Build history of the part. All positions in model axes, mm. A direction names the side the tool comes from. Coordinates: 2 decimals unless noted, no trailing zeros. Loops run counter-clockwise (first coordinate to the right, second up) from the corner with the lowest first, then second, coordinate; pieces in that order, holes last.
Item 1: Flat gauge pins, fed straight in: pin 1 (3 mm diameter, centred on y = 12.5, z = 1, fed in from +X); pin 2 (11.5 mm diameter, centred on x = 0, y = 15, fed in from +Z); pin 3 (1.5 mm diameter, centred on x = 18.5, z = 4.5, fed in from -Y); pin 4 (3 mm diameter, centred on x = -9.5, z = 2.5, fed in from +Y). Where does each tip first touch, or does it go through?
Item 2: Cut at D-D (x = -23.5). List the corners of the cut face in (y, z).
Item 3: 3-axis set-ups, long thin cutter, end or side, ignore diameter. For faces 1 (the face through (0, 0, 0)), 2 (the face through (26, 0, 2)): which of +Z, -Z, +X, -X, +Y, -Y reach the whole face in a straight line?
Item 4: Drill centre lines: line 1 along Y through (x, z) = (0, 2); line 2 along X through (y, z) = (-17, 3.45); line 3 along Y through (x, z) = (-3.5, 0.35). Where is each one in solid material? Low to high.
Item 5: Cut at A-A (z = 2.15). List the corners of the cut face in (x, y), and give its area (3 significant figures).
Item 6: Cut at B-B (x = 0). List the corners of the cut face in (y, z), and give its area (3 significant figures).
Item 7: Cut at C-C (y = 0). List the corners of the cut face in (x, z), and give its area (4 significant figures).
Item 8: Mould opens along Y. For faces 3 (the face through (0, 0, 5)), 4 (the face through (-29.97, -1.32, 2.46)), 5 (the face through (15.76, -18.41, 2.46)) say: released by +Y, released by -Y, zero draft, split by the parting line, or undercut.
Autodesk Fusion 360 part; units mm, degrees
sketch "Sketch1" plane through (0, 0, 0) normal (0, 0, 1) x (1, 0, 0)
  circle A0 centre (0, -15) radius 5
  circle A1 centre (0, 15) radius 5
  line L0 (26.5, 0) -> (27.807, 0) construction
  circle A2 centre (0, 0) radius 30
  line L1 (22.25, 0) -> (27.7377, 0) construction
  arc A3 (18.3848, 18.3848) -> (15.7331, 15.7331) centre (17.059, 17.059) ccw
  arc A4 (-15.7331, 15.7331) -> (-18.3848, 18.3848) centre (-17.059, 17.059) ccw
  arc A5 (15.7331, -15.7331) -> (18.3848, -18.3848) centre (17.059, -17.059) ccw
  arc A6 (-18.3848, -18.3848) -> (-15.7331, -15.7331) centre (-17.059, -17.059) ccw
  arc A7 (-15.7331, 15.7331) -> (-15.7331, -15.7331) centre (0, 0) ccw
  arc A8 (15.7331, -15.7331) -> (15.7331, 15.7331) centre (0, 0) ccw
  arc A9 (-18.3848, 18.3848) -> (-18.3848, -18.3848) centre (0, 0) ccw
  arc A10 (18.3848, -18.3848) -> (18.3848, 18.3848) centre (0, 0) ccw
  dimension "d4" = 15
  dimension "d5" = 10
  dimension "d11" = 60
  dimension "d12" = 52
  dimension "d16" = 44.5
  dimension "d17" = 3.75
extrude "Extrude1" add sketch "Sketch1" along normal blind 5
Filled sheet:
1. pin 1: stops at x = 27.91
1. pin 2: stops at z = 5
1. pin 3: stops at y = -24.19
1. pin 4: stops at y = 28.91
2. outline: (-18.65, 0) - (-11.12, 0) - (-11.12, 5) - (-18.65, 5) - close; (11.12, 0) - (18.65, 0) - (18.65, 5) - (11.12, 5) - close
3. face 1: -Z, +X, -X, +Y, -Y
3. face 2: +Z, -Z
4. line 1: y = -30 to -20, -10 to 10, 20 to 30
4. line 2: x = -24.72 to -19.67, -15.18 to -4.58, 4.58 to 15.18, 19.67 to 24.72
4. line 3: y = -29.8 to -18.57, -11.43 to 11.43, 18.57 to 29.8
5. outline: circle Ø60 at (0, 0); hole (-18.38, -18.38) arc R1.88 ccw to (-15.73, -15.73) arc R22.25 cw to (-15.73, 15.73) arc R1.88 ccw to (-18.38, 18.38) arc R26 ccw to start; hole circle Ø10 at (0, -15); hole circle Ø10 at (0, 15); hole (15.73, -15.73) arc R1.88 ccw to (18.38, -18.38) arc R26 ccw to (18.38, 18.38) arc R1.88 ccw to (15.73, 15.73) arc R22.25 cw to start
5. area: 2,360 mm2
6. outline: (-30, 0) - (-20, 0) - (-20, 5) - (-30, 5) - close; (-10, 0) - (10, 0) - (10, 5) - (-10, 5) - close; (20, 0) - (30, 0) - (30, 5) - (20, 5) - close
6. area: 200 mm2
7. outline: (-30, 0) - (-26, 0) - (-26, 5) - (-30, 5) - close; (-22.25, 0) - (22.25, 0) - (22.25, 5) - (-22.25, 5) - close; (26, 0) - (30, 0) - (30, 5) - (26, 5) - close
7. area: 262.5 mm2
8. face 3: zero draft
8. face 4: split by the parting line
8. face 5: undercut
